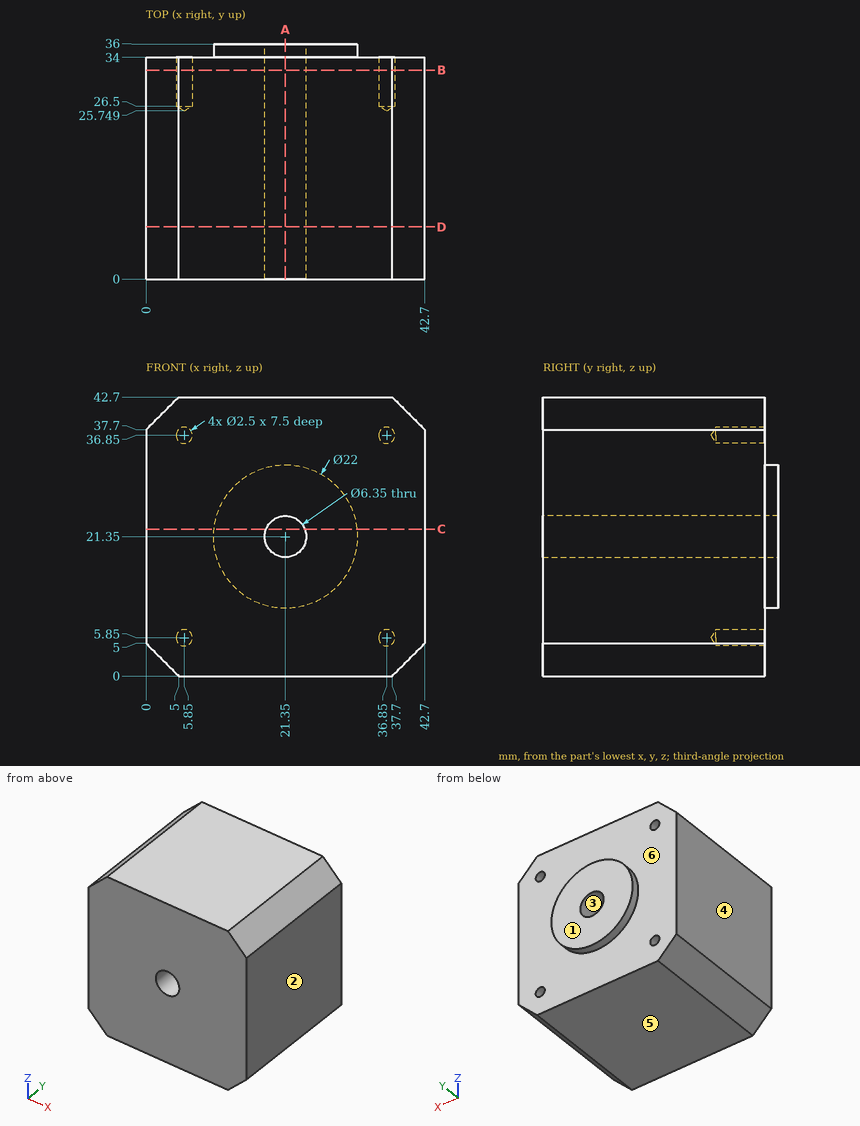
Verification items for this drawing (mm, ordinates from the low corner). A direction names the side the tool comes from. Round coordinates to 2 decimals unless told otherwise and drop trailing zeros. Write each loop counter-clockwise with the first axis right and the second up, starting at its lowest first coordinate (ties: lowest second). Pieces come first, ordered by that corner, then holes. Notation, with made-up numbers: (5, 64) - (64, 64) arc R19 cw to (64, 99) - close; hole circle Ø7 at (-38.5, 38). An arc over 180 degrees is marked (long way). One line per item, written item: value.
1. Cross-section at A-A on x = 21.35. Record the boundary of the cut face in (y, z) (3 decimals), and give its area (3 significant figures).
The answers:
outline: (0, 0) - (34, 0) - (34, 10.35) - (36, 10.35) - (36, 18.175) - (0, 18.175) - close; (0, 24.525) - (36, 24.525) - (36, 32.35) - (34, 32.35) - (34, 42.7) - (0, 42.7) - close
area: 1,270 mm^2
2. Set-up check for the marked faces 5 and 6: record each of +Z, -Z, +X, -X, +Y, -Y from which the full face is reachable in a straight line by a thin tool's end or side.
The answers:
face 5: -Z, +X, -X, +Y, -Y
face 6: +Y
3. Scan lines: L1, parallel to Z at x = 36.85, y = 29.5; L2, parallel to Z at x = 36, y = 31; L3, parallel to Y at x = 21, z = 3. Record each from-to range of solid material in increasing order.
The answers:
L1: z = 0 to 4.6, 7.1 to 35.6, 38.1 to 42.7
L2: z = 0 to 4.93, 6.77 to 35.93, 37.77 to 42.7
L3: y = 0 to 34
4. Mould release check, pull along X, two halves, no side actions. Record for the marked faces 1, 2, 3 and 4: released by +X, released by -X, zero draft, split by the parting line, or undercut.
The answers:
face 1: zero draft
face 2: released by +X
face 3: undercut
face 4: released by -X
5. Cross-section at D-D on y = 8. Record the boundary of the cut face in (x, z) (3 decimals).
The answers:
outline: (0, 5) - (5, 0) - (37.7, 0) - (42.7, 5) - (42.7, 37.7) - (37.7, 42.7) - (5, 42.7) - (0, 37.7) - close; hole circle Ø6.35 at (21.35, 21.35)
6. Cross-section at B-B on y = 32. Record the boundary of the cut face in (x, z) (3 decimals).
The answers:
outline: (0, 5) - (5, 0) - (37.7, 0) - (42.7, 5) - (42.7, 37.7) - (37.7, 42.7) - (5, 42.7) - (0, 37.7) - close; hole circle Ø2.5 at (5.85, 5.85); hole circle Ø2.5 at (5.85, 36.85); hole circle Ø6.35 at (21.35, 21.35); hole circle Ø2.5 at (36.85, 5.85); hole circle Ø2.5 at (36.85, 36.85)
7. Depth check by flat-ended pin: pin 1 Ø4 at (x, z) = (5.85, 5.85) entering from +Y; pin 2 Ø5.5 at (x, z) = (21.35, 21.35) entering from +Y. Enter the tip coordinate at first touch or a pass-through.
The answers:
pin 1: stops at y = 34
pin 2: passes through
8. Cross-section at C-C on z = 22.5. Record the boundary of the cut face in (x, y), and give its area (3 significant figures).
The answers:
outline: (0, 0) - (18.39, 0) - (18.39, 36) - (10.41, 36) - (10.41, 34) - (0, 34) - close; (24.31, 0) - (42.7, 0) - (42.7, 34) - (32.29, 34) - (32.29, 36) - (24.31, 36) - close
area: 1,280 mm^2
